Can you work these out from the model? Positions are in its coordinate system, mm. Coordinates: 2 decimals unless noted, no trailing zeros. Order: outer loops, then holes, each group sorted by start corner. A loop starts at its lowest first (then second) coordinate and runs counter-clockwise, first axis right, second up. Notation, with made-up numbers: M 47,82 L 57,82 A21 ccw 57,99 Z; hole C 86.5,-22.5 d3. An arc over 180 degrees is marked long. Answer as a JSON object with one key per item and string values.
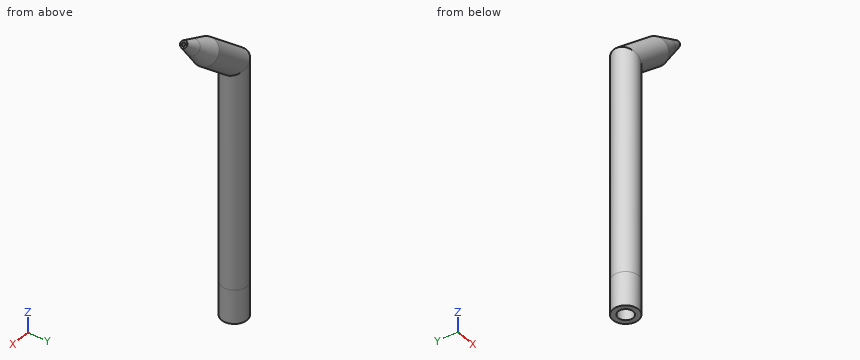
from build123d import *

# Parameters (mm, degrees)
SKETCH_1_R      = 7.5
SKETCH_1_R_2    = 4.5
EXTRUDE_1_DEPTH = 100
SKETCH_3_R      = 7.5
SKETCH_3_R_2    = 4.5
EXTRUDE_START   = 20
SKETCH_6_R      = 7.5
SKETCH_6_R_2    = 4.5
EXTRUDE_2_DEPTH = 20


with BuildPart() as part:
    # 草图1 → 凸台-拉伸1 (new body)
    with BuildSketch(Plane.XY):
        Circle(SKETCH_1_R)
        Circle(SKETCH_1_R_2, mode=Mode.SUBTRACT)
    extrude(amount=EXTRUDE_1_DEPTH)

    # 扫描1: sweep along a path in 草图2
    with BuildLine(Plane(origin=(0, 0, 0), x_dir=(1, 0, 0), z_dir=(0, 1, 0))) as sweep_1_path:
        Line((0, -100), (0, -130))
        Line((0, -130), (22.981333294, -149.283628291))
    # 草图3 → 扫描1 (sweep)
    with BuildSketch(Plane.XY.offset(100)):
        Circle(SKETCH_3_R)
        Circle(SKETCH_3_R_2, mode=Mode.SUBTRACT)
    sweep(path=sweep_1_path.line, transition=Transition.RIGHT)

    # 草图5 → 旋转1 (revolve)
    with BuildSketch(Plane(origin=(0, 0, 0), x_dir=(1, 0, 0), z_dir=(0, 1, 0)), mode=Mode.PRIVATE) as revolve_1_sk:
        Polygon((27.802240366, -143.538294967), (25.873877537, -145.836428297), (33.630329642, -156.91378991), (40.52252136, -162.697025438), (41.16530897, -161.930980995), (35.728697758, -154.448127615), align=None)
    revolve(revolve_1_sk.sketch.rotate(Axis((0, 0, 130), (0.7660444431189799, 0, 0.6427876096865373)), 180), axis=Axis((0, 0, 130), (0.7660444431189799, 0, 0.6427876096865373)))

    # 草图6 → 凸台-拉伸2 (add)
    with BuildSketch(Plane(origin=(0, 0, 0), x_dir=(-1, 0, 0), z_dir=(0, 0, -1)).offset(EXTRUDE_START)):
        Circle(SKETCH_6_R)
        Circle(SKETCH_6_R_2, mode=Mode.SUBTRACT)
    extrude(amount=-EXTRUDE_2_DEPTH)


solid = part.part
Item 1: Please list where these lines run through material, in increasing order: line 1 (X direction, y = 0, z = -9.5); line 2 (X direction, y = 2.5, z = 39).
Answers follow:
{"line 1": "x = -7.5 to -4.5, 4.5 to 7.5", "line 2": "x = -7.07 to -3.74, 3.74 to 7.07"}
Item 2: I want a section at A-A, the plane z = 27.5. Write out the boundary of the cut face in (x, y), plus the area to 3 significant figures.
Answers follow:
{"outline": "C 0,0 d15; hole C 0,0 d9", "area": "113 mm^2"}
Item 3: I'm going to push flat-ended pins straight in: pin 1 (8 mm diameter, centred on x = 0, y = 0, fed in from -Z); pin 2 (5 mm diameter, centred on x = 31.5, y = -4.5, fed in from -Z); pin 3 (1 mm diameter, centred on y = -3.5, z = 30, fed in from -X). Where does each tip first touch, or does it pass through?
Answers follow:
{"pin 1": "stops at z = 132.06", "pin 2": "stops at z = 147.04", "pin 3": "stops at x = -6.87"}
